Geometry check sheet. Reference: the model listing, model coordinates, mm. Round coordinates to 2 decimals unless told otherwise and drop trailing zeros. Return JSON: item names as keys, results as strings. Group by question number.
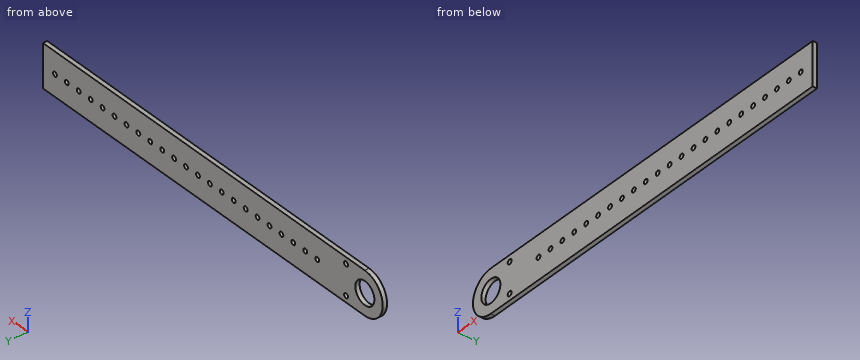
Autodesk Inventor part; units mm, degrees
ref_plane "YZ Plane" through (0, 0, 0) normal (1, 0, 0) x (0, 1, 0)
ref_plane "XZ Plane" through (0, 0, 0) normal (0, 1, 0) x (-1, 0, 0)
ref_plane "XY Plane" through (0, 0, 0) normal (0, 0, 1) x (1, 0, 0)
sketch "スケッチ1" plane through (0, 0, 0) normal (0, 1, 0) x (-1, 0, 0)
  line L0 (0, 0) -> (-287.5, 0)
  line L1 (-287.5, 0) -> (-287.5, -30)
  line L2 (-287.5, -30) -> (0, -30)
  line L3 (0, -30) -> (0, 0)
  arc A0 (-17.5, -30) -> (-17.5, 0) centre (-17.5, -15) ccw
  dimension "d0" = 287.5
  dimension "d1" = 30
  dimension "d43" = 17.5
extrude "押し出し1" add sketch "スケッチ1" along normal blind 3 contours A0 L2 L1 L0
sketch "スケッチ2" plane through (0, 3, 0) normal (0, 1, 0) x (1, 0, 0)
  arc A0 (17.5, 30) -> (17.5, 0) centre (17.5, 15) ccw
  line L0 (287.5, 30) -> (17.5, 30)
  point P0 (0, 0)
  point P1 (2.5, 15)
hole "穴1" at (17.5, 3, -15) direction (0, -1, 0) diameter 16 end through all
sketch "スケッチ3" plane through (0, 3, 0) normal (0, 1, 0) x (1, 0, 0)
  line L0 (287.5, 0) -> (287.5, 30)
  arc A0 (17.5, 30) -> (17.5, 0) centre (17.5, 15) ccw construction
  line L1 (17.5, 15) -> (287.5, 15) construction
  line L2 (287.5, 0) -> (287.5, 30) construction
  point P0 (0, 0)
  point P1 (57.5, 15)
  point P2 (67.5, 15)
  point P3 (77.5, 15)
  point P4 (87.5, 15)
  point P5 (97.5, 15)
  point P6 (107.5, 15)
  point P7 (117.5, 15)
  point P8 (127.5, 15)
  point P9 (137.5, 15)
  point P10 (147.5, 15)
  point P11 (157.5, 15)
  point P12 (167.5, 15)
  point P13 (177.5, 15)
  point P14 (187.5, 15)
  point P15 (197.5, 15)
  point P16 (207.5, 15)
  point P17 (217.5, 15)
  point P18 (227.5, 15)
  point P19 (237.5, 15)
  point P20 (247.5, 15)
  point P21 (257.5, 15)
  point P22 (267.5, 15)
  point P23 (277.5, 15)
  dimension "d108" = 40
  dimension "d111" = 10
sketch "スケッチ8" plane through (0, 3, 0) normal (0, 1, 0) x (1, 0, 0)
  arc A0 (17.5, 30) -> (17.5, 0) centre (17.5, 15) ccw
  line L0 (2.5, 15) -> (40.1182, 15)
  line L1 (17.5, 0) -> (287.5, 0)
  line L2 (2.5, 15) -> (302.5, 15) construction
  circle A1 centre (17.5, 15) radius 8 construction
  point P0 (0, 0)
  point P1 (33.3, 4.5)
  point P2 (33.3, 25.5)
  dimension "d85" = 10.5
  dimension "d86" = 10.5
  dimension "d123" = 15.8
  dimension "d124" = 15.8
hole "穴6" at (33.3, 3, -4.5) at (33.3, 3, -25.5) direction (0, -1, 0) diameter 3.3 end through all
hole "穴7" at (57.5, 3, -15) at (67.5, 3, -15) at (77.5, 3, -15) at (87.5, 3, -15) at (97.5, 3, -15) at (107.5, 3, -15) at (117.5, 3, -15) at (127.5, 3, -15) at (137.5, 3, -15) at (147.5, 3, -15) at (157.5, 3, -15) at (167.5, 3, -15) at (177.5, 3, -15) at (187.5, 3, -15) at (197.5, 3, -15) at (207.5, 3, -15) at (217.5, 3, -15) at (227.5, 3, -15) at (237.5, 3, -15) at (247.5, 3, -15) at (257.5, 3, -15) at (267.5, 3, -15) at (277.5, 3, -15) direction (0, -1, 0) diameter 3.2 end through all
properties part number "shoulder1_upper_plate" material "アルミニウム 5052"
Q1. Section check A-A on y = 0.7. Count the separate pieces of the cut face and the enclosed holes in it, plus the area to 3 significant figures.
Q2. Material ranges on line 1 along Z through (x, y) = (137.5, 1.05); line 2 along Z through (x, y) = (33.3, 1.05); line 3 along X through (y, z) = (1.9, -21.25), recorded low to high.
Q3. Depth check by flat-ended pin: pin 1 Ø9.5 at (x, z) = (17.5, -15) entering from +Y; pin 2 Ø4.5 at (x, z) = (33.3, -25.5) entering from +Y. Enter the tip coordinate at first touch or a pass-through.
Geometry check:
{
 "1": {"separate pieces": "1", "enclosed holes": "26", "area": "8,050 mm^2"},
 "2": {"line 1": "z = -30 to -16.6, -13.4 to 0", "line 2": "z = -30 to -27.15, -23.85 to -6.15, -2.85 to 0", "line 3": "x = 3.86 to 12.51, 22.49 to 287.5"},
 "3": {"pin 1": "passes through", "pin 2": "stops at y = 3"}
}
